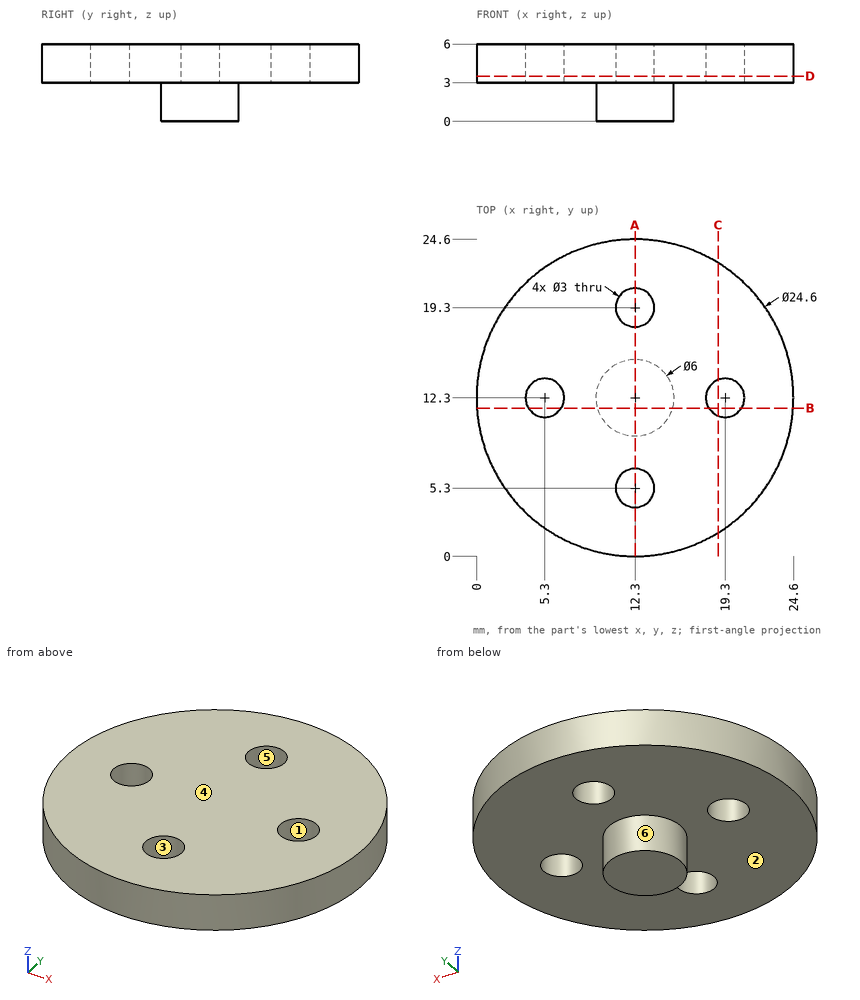
Geometry: see drawing. Coordinates: mm, zero at the bounding-box minimum. A direction names the side the tool comes from. Round coordinates to 2 decimals unless told otherwise and drop trailing zeros. Loops run counter-clockwise (first coordinate to the right, second up) from the corner with the lowest first, then second, coordinate; pieces in that order, holes last. Notation, with made-up numbers: (82.25, 74) - (131.25, 74) arc R23 ccw to (131.25, 96) - close; hole circle Ø5 at (3.5, -7.5). An arc over 180 degrees is marked (long way). Write item = value, one per line. Start each with the question number.
(1) Ray query, line 1 along Y through (x, z) = (12.3, 5.4); line 2 along Z through (x, y) = (16.75, 10.75); line 3 along X through (y, z) = (20.25, 5). Return the intervals inside material, ascending. Write a range as from..to.
(2) Section query D-D, the plane z = 3.5. Output: boundary loops of the cut face in (x, y).
(3) Section query B-B, the plane y = 11.5. Output: boundary loops of the cut face in (x, z), plus the area to 3 significant figures.
(4) Pin query (flat end, axial travel): pin 1 (4 mm diameter, centred on x = 12.3, y = 19.3, fed in from -Z); pin 2 (3 mm diameter, centred on y = 15.5, z = 4.5, fed in from -X); pin 3 (1 mm diameter, centred on x = 17, z = 1, fed in from -Y). Return the tip coordinate at first contact, or that it passes through.
(5) Section query C-C, the plane x = 18.75. Output: boundary loops of the cut face in (y, z).
(6) Set-up query: the marked faces 1 and 2. Return all of +Z, -Z, +X, -X, +Y, -Y with unobstructed straight access to the full face (end or side cutting, diameter ignored); none if empty.
(7) Section query A-A, the plane x = 12.3. Output: boundary loops of the cut face in (y, z).
(8) Pull-direction query (X, two-part tool) for the marked faces 3, 4, 5 and 6; classes: +X half, -X half, draft (parallel to the pull), parting line (faces both ways), or undercut.
Conclusion:
q1.line_1 = 0..3.8, 6.8..17.8, 20.8..24.6
q1.line_2 = 3..6
q1.line_3 = 2.91..11.14, 13.46..21.69
q2.outline = circle Ø24.6 at (12.3, 12.3); hole circle Ø3 at (5.3, 12.3); hole circle Ø3 at (12.3, 5.3); hole circle Ø3 at (12.3, 19.3); hole circle Ø3 at (19.3, 12.3)
q3.outline = (0.03, 3) - (4.03, 3) - (4.03, 6) - (0.03, 6) - close; (6.57, 3) - (9.41, 3) - (9.41, 0) - (15.19, 0) - (15.19, 3) - (18.03, 3) - (18.03, 6) - (6.57, 6) - close; (20.57, 3) - (24.57, 3) - (24.57, 6) - (20.57, 6) - close
q3.area = 75.8 mm2
q4.pin_1 = 3
q4.pin_2 = 0.12
q4.pin_3 = through
q5.outline = (1.83, 3) - (10.9, 3) - (10.9, 6) - (1.83, 6) - close; (13.7, 3) - (22.77, 3) - (22.77, 6) - (13.7, 6) - close
q6.face_1 = +Z, -Z
q6.face_2 = -Z
q7.outline = (0, 3) - (3.8, 3) - (3.8, 6) - (0, 6) - close; (6.8, 3) - (9.3, 3) - (9.3, 0) - (15.3, 0) - (15.3, 3) - (17.8, 3) - (17.8, 6) - (6.8, 6) - close; (20.8, 3) - (24.6, 3) - (24.6, 6) - (20.8, 6) - close
q8.face_3 = undercut
q8.face_4 = draft
q8.face_5 = undercut
q8.face_6 = parting line
